Answer from the drawing. Dimensions are ordinates in mm from the lowest x, y and z of the part. A direction names the side the tool comes from. Coordinates: 2 decimals unless noted, no trailing zeros. Order: outer loops, then holes, each group sorted by start corner. A loop starts at its lowest first (then second) coordinate and runs counter-clockwise, first axis right, second up. Notation, with made-up numbers: (-21, -33) - (32, -33) arc R16 ccw to (32, -17) - close; hole circle Ø3 at (22, 30.5). An arc over 180 degrees is marked (long way). Use CSV: the item, a comma, the result in double quotes. Start each with the question number.
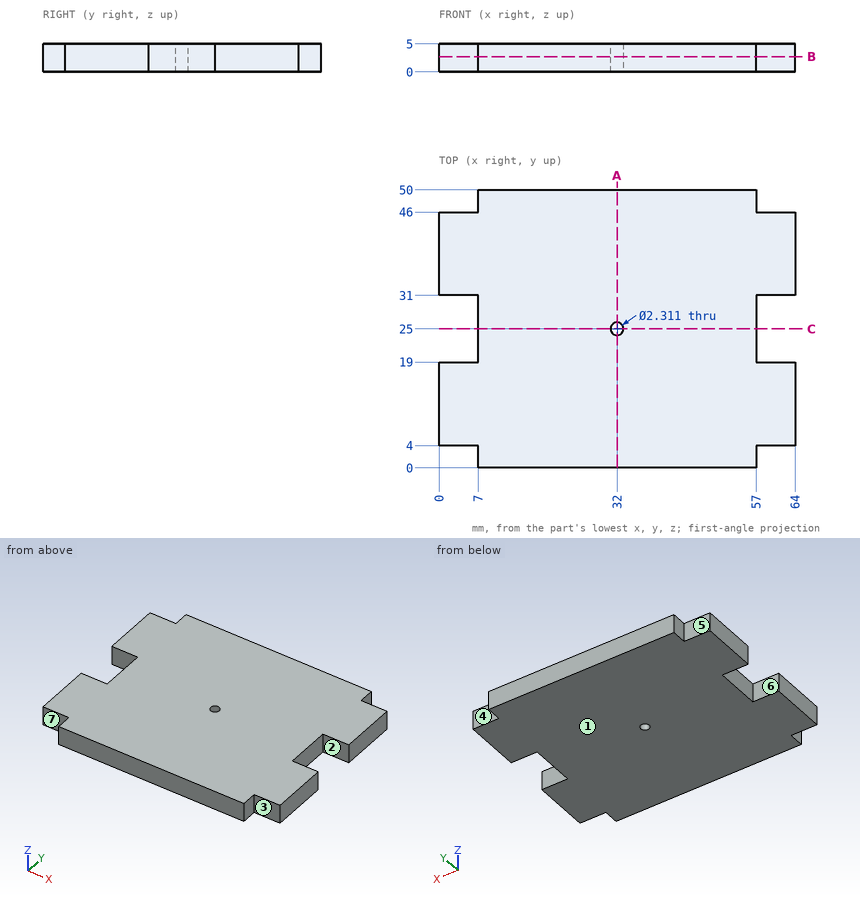
1) Flat-ended cylindrical pins translate along their axes: P1, Ø3, axis at x = 24.5, z = 4, coming from the -Y side; P2, Ø2.5, axis at y = 26, z = 1.5, coming from the -X side; P3, Ø1.2, axis at y = 47.5, z = 2.5, coming from the +X side; P4, Ø1.5, axis at x = 61.5, z = 1.5, coming from the -Y side. Find the tip coordinate at first contact, or state that the pin passes through.
2) For a pull along Y with two mould halves and no side action, classify the marked faces 1, 2 and 3 as +Y half, -Y half, draft (parallel to the pull), parting line (faces both ways), or undercut.
3) The part is cut by section A-A on x = 32. Determine the outline of the cut face in (y, z) (1 decimal).
4) The part is cut by section C-C on y = 25. Determine the outline of the cut face in (x, z) (1 decimal).
5) Straight lines are drawn through the part: line 1 (Y direction, x = 32, z = 3.9) (1 decimal); line 2 (X direction, y = 27.5, z = 4.3); line 3 (Y direction, x = 6, z = 0.3). For each, find the intervals that lie inside material, in ascending order. Write a range as [from, to].
6) For the marked faces 4, 5, 6 and 7, determine the directions among +Z, -Z, +X, -X, +Y, -Y from which every point of the face is accessible in a straight line to the end or side of a thin tool.
7) The part is cut by section B-B on z = 2.75. Determine the outline of the cut face in (x, y) (1 decimal).
Answer key:
1,P1,"y = 0"
1,P2,"x = 7"
1,P3,"x = 57"
1,P4,"y = 4"
2,face 1,"draft"
2,face 2,"undercut"
2,face 3,"-Y half"
3,outline,"(0, 0) - (23.8, 0) - (23.8, 5) - (0, 5) - close; (26.2, 0) - (50, 0) - (50, 5) - (26.2, 5) - close"
4,outline,"(7, 0) - (30.8, 0) - (30.8, 5) - (7, 5) - close; (33.2, 0) - (57, 0) - (57, 5) - (33.2, 5) - close"
5,line 1,"[0, 23.8], [26.2, 50]"
5,line 2,"[7, 57]"
5,line 3,"[4, 19], [31, 46]"
6,face 4,"+Z, -Z, +X, +Y"
6,face 5,"+Z, -Z, -X, +Y"
6,face 6,"+Z, -Z, -X"
6,face 7,"+Z, -Z, -X, -Y"
7,outline,"(0, 4) - (7, 4) - (7, 0) - (57, 0) - (57, 4) - (64, 4) - (64, 19) - (57, 19) - (57, 31) - (64, 31) - (64, 46) - (57, 46) - (57, 50) - (7, 50) - (7, 46) - (0, 46) - (0, 31) - (7, 31) - (7, 19) - (0, 19) - close; hole circle Ø2.3 at (32, 25)"
